from build123d import *

# Parameters (mm, degrees)
SKETCH_2_W             = 126
SKETCH_2_H             = 22
SKETCH_2_R             = 1.7
SM_BASE_FLANGE_1_DEPTH = 2.5
OTHER_START            = -15.764824005
OTHER_1_DEPTH          = 22
OTHER_START_2          = -11.014823905
OTHER_1_2_DEPTH        = 12.4999998
OTHER_1_3_DEPTH        = 1.3499999
OTHER_START_3          = 4.885176095
OTHER_1_4_DEPTH        = 1.3499999
OTHER_START_4          = -14.414824105
OTHER_1_5_DEPTH        = 19.3000002
OTHER_START_5          = -51.7366
OTHER_1_6_OUTLINE_R    = 1.7
OTHER_1_6_DEPTH        = 103.4732
CUT_EXTRUDE_1_DEPTH    = 57.025302757


with BuildPart() as part:
    # 基体-法兰1: sheet metal written as solids
    # Sketch 2 → 基体-法兰1 (new body)
    with BuildSketch(Plane(origin=(0, 0, 0), x_dir=(1, 0, 0), z_dir=(0, 1, 0))):
        with Locations((0, 4.764824005)):
            Rectangle(SKETCH_2_W, SKETCH_2_H)
        with Locations(Location((57.5, 12.714824005, 0), (0, 0, 270))):
            Circle(SKETCH_2_R, mode=Mode.SUBTRACT)
        with Locations(Location((57.5, -3.185175995, 0), (0, 0, 270))):
            Circle(SKETCH_2_R, mode=Mode.SUBTRACT)
        with Locations(Location((-57.5, -3.185175995, 0), (0, 0, 90))):
            Circle(SKETCH_2_R, mode=Mode.SUBTRACT)
        with Locations(Location((-57.5, 12.714824005, 0), (0, 0, 90))):
            Circle(SKETCH_2_R, mode=Mode.SUBTRACT)
    extrude(amount=-SM_BASE_FLANGE_1_DEPTH)

    # Other 1: read off the stored shape, not the designer's step
    # Other 1 outline → Other 1 (cut)
    with BuildSketch(Plane.XY.offset(OTHER_START)):
        with BuildLine():
            Line((-63, -2.5), (-48.5, -2.5))
            ThreePointArc((-48.5, -2.5), (-50.511404982, -1.799110859), (-51.651666226, 0))
            Line((-51.651666226, 0), (-63, 0))
            Line((-63, 0), (-63, -2.5))
        make_face()
        with BuildLine():
            ThreePointArc((51.651666226, 0), (50.511404982, -1.799110859), (48.5, -2.5))
            Line((48.5, -2.5), (63, -2.5))
            Line((63, -2.5), (63, 0))
            Line((63, 0), (51.651666226, 0))
        make_face()
    extrude(amount=OTHER_1_DEPTH, mode=Mode.SUBTRACT)

    # Other 1 2 outline → Other 1 2 (add)
    with BuildSketch(Plane.XY.offset(OTHER_START_2)):
        with BuildLine():
            ThreePointArc((-51.7366, 0.7366), (-51.715296446, 0.365859759), (-51.651666226, 0))
            Line((-51.651666226, 0), (-48.5, 0))
            ThreePointArc((-48.5, 0), (-49.020854855, 0.215745145), (-49.2366, 0.7366))
            Line((-49.2366, 0.7366), (-49.2366, 12.116056017))
            Line((-49.2366, 12.116056017), (-51.7366, 12.116056017))
            Line((-51.7366, 12.116056017), (-51.7366, 0.7366))
        make_face()
        with BuildLine():
            Line((48.5, 0), (51.651666226, 0))
            ThreePointArc((51.651666226, 0), (51.715296446, 0.365859759), (51.7366, 0.7366))
            Line((51.7366, 0.7366), (51.7366, 12.116056017))
            Line((51.7366, 12.116056017), (49.2366, 12.116056017))
            Line((49.2366, 12.116056017), (49.2366, 0.7366))
            ThreePointArc((49.2366, 0.7366), (49.020854855, 0.215745145), (48.5, 0))
        make_face()
    extrude(amount=OTHER_1_2_DEPTH)

    # Other 1 3 outline → Other 1 3 (add)
    with BuildSketch(Plane.XY.offset(OTHER_START)):
        with BuildLine():
            ThreePointArc((-51.7366, 0.7366), (-51.715296446, 0.365859759), (-51.651666226, 0))
            Line((-51.651666226, 0), (-48.5, 0))
            ThreePointArc((-48.5, 0), (-49.020854855, 0.215745145), (-49.2366, 0.7366))
            Line((-49.2366, 0.7366), (-49.2366, 12.116056017))
            Line((-49.2366, 12.116056017), (-51.7366, 12.116056017))
            Line((-51.7366, 12.116056017), (-51.7366, 0.7366))
        make_face()
        with BuildLine():
            Line((48.5, 0), (51.651666226, 0))
            ThreePointArc((51.651666226, 0), (51.715296446, 0.365859759), (51.7366, 0.7366))
            Line((51.7366, 0.7366), (51.7366, 12.116056017))
            Line((51.7366, 12.116056017), (49.2366, 12.116056017))
            Line((49.2366, 12.116056017), (49.2366, 0.7366))
            ThreePointArc((49.2366, 0.7366), (49.020854855, 0.215745145), (48.5, 0))
        make_face()
    extrude(amount=OTHER_1_3_DEPTH)

    # Other 1 4 outline → Other 1 4 (add)
    with BuildSketch(Plane.XY.offset(OTHER_START_3)):
        with BuildLine():
            ThreePointArc((-51.7366, 0.7366), (-51.715296446, 0.365859759), (-51.651666226, 0))
            Line((-51.651666226, 0), (-48.5, 0))
            ThreePointArc((-48.5, 0), (-49.020854855, 0.215745145), (-49.2366, 0.7366))
            Line((-49.2366, 0.7366), (-49.2366, 12.116056017))
            Line((-49.2366, 12.116056017), (-51.7366, 12.116056017))
            Line((-51.7366, 12.116056017), (-51.7366, 0.7366))
        make_face()
        with BuildLine():
            Line((48.5, 0), (51.651666226, 0))
            ThreePointArc((51.651666226, 0), (51.715296446, 0.365859759), (51.7366, 0.7366))
            Line((51.7366, 0.7366), (51.7366, 12.116056017))
            Line((51.7366, 12.116056017), (49.2366, 12.116056017))
            Line((49.2366, 12.116056017), (49.2366, 0.7366))
            ThreePointArc((49.2366, 0.7366), (49.020854855, 0.215745145), (48.5, 0))
        make_face()
    extrude(amount=OTHER_1_4_DEPTH)

    # Other 1 5 outline → Other 1 5 (add)
    with BuildSketch(Plane.XY.offset(OTHER_START_4)):
        with BuildLine():
            ThreePointArc((49.2366, 0.7366), (49.020854855, 0.215745145), (48.5, 0))
            Line((48.5, 0), (51.651666226, 0))
            ThreePointArc((51.651666226, 0), (51.715296446, 0.365859759), (51.7366, 0.7366))
            Line((51.7366, 0.7366), (51.7366, 12.116056017))
            Line((51.7366, 12.116056017), (49.2366, 12.116056017))
            Line((49.2366, 12.116056017), (49.2366, 0.7366))
        make_face()
        with BuildLine():
            ThreePointArc((-51.7366, 0.7366), (-51.715296446, 0.365859759), (-51.651666226, 0))
            Line((-51.651666226, 0), (-48.5, 0))
            ThreePointArc((-48.5, 0), (-49.020854855, 0.215745145), (-49.2366, 0.7366))
            Line((-49.2366, 0.7366), (-49.2366, 12.116056017))
            Line((-49.2366, 12.116056017), (-51.7366, 12.116056017))
            Line((-51.7366, 12.116056017), (-51.7366, 0.7366))
        make_face()
    extrude(amount=OTHER_1_5_DEPTH)

    # Other 1 6 outline → Other 1 6 (cut)
    with BuildSketch(Plane.YZ.offset(OTHER_START_5)):
        with Locations((6.616056017, -12.714824005)):
            Circle(OTHER_1_6_OUTLINE_R)
        with Locations((6.616056017, 3.185175995)):
            Circle(OTHER_1_6_OUTLINE_R)
    extrude(amount=OTHER_1_6_DEPTH, mode=Mode.SUBTRACT)

    # 草图8 → 切除-拉伸1 (cut, through all)
    with BuildSketch(Plane.XZ.offset(2.5)):
        with BuildLine():
            Line((-8, -3.764824005), (8, -3.764824005))
            ThreePointArc((8, -3.764824005), (9, -4.764824005), (8, -5.764824005))
            Line((8, -5.764824005), (-8, -5.764824005))
            ThreePointArc((-8, -5.764824005), (-9, -4.764824005), (-8, -3.764824005))
        make_face()
        with BuildLine():
            Line((-38, -3.764824005), (-22, -3.764824005))
            ThreePointArc((-22, -3.764824005), (-21, -4.764824005), (-22, -5.764824005))
            Line((-22, -5.764824005), (-38, -5.764824005))
            ThreePointArc((-38, -5.764824005), (-39, -4.764824005), (-38, -3.764824005))
        make_face()
        with BuildLine():
            Line((22, -3.764824005), (38, -3.764824005))
            ThreePointArc((38, -3.764824005), (39, -4.764824005), (38, -5.764824005))
            Line((38, -5.764824005), (22, -5.764824005))
            ThreePointArc((22, -5.764824005), (21, -4.764824005), (22, -3.764824005))
        make_face()
        with BuildLine():
            Line((-8, -11.764824005), (8, -11.764824005))
            ThreePointArc((8, -11.764824005), (9, -12.764824005), (8, -13.764824005))
            Line((8, -13.764824005), (-8, -13.764824005))
            ThreePointArc((-8, -13.764824005), (-9, -12.764824005), (-8, -11.764824005))
        make_face()
        with BuildLine():
            Line((-38, -11.764824005), (-22, -11.764824005))
            ThreePointArc((-22, -11.764824005), (-21, -12.764824005), (-22, -13.764824005))
            Line((-22, -13.764824005), (-38, -13.764824005))
            ThreePointArc((-38, -13.764824005), (-39, -12.764824005), (-38, -11.764824005))
        make_face()
        with BuildLine():
            Line((22, -11.764824005), (38, -11.764824005))
            ThreePointArc((38, -11.764824005), (39, -12.764824005), (38, -13.764824005))
            Line((38, -13.764824005), (22, -13.764824005))
            ThreePointArc((22, -13.764824005), (21, -12.764824005), (22, -11.764824005))
        make_face()
        with BuildLine():
            Line((-8, 4.235175995), (8, 4.235175995))
            ThreePointArc((8, 4.235175995), (9, 3.235175995), (8, 2.235175995))
            Line((8, 2.235175995), (-8, 2.235175995))
            ThreePointArc((-8, 2.235175995), (-9, 3.235175995), (-8, 4.235175995))
        make_face()
        with BuildLine():
            Line((-38, 4.235175995), (-22, 4.235175995))
            ThreePointArc((-22, 4.235175995), (-21, 3.235175995), (-22, 2.235175995))
            Line((-22, 2.235175995), (-38, 2.235175995))
            ThreePointArc((-38, 2.235175995), (-39, 3.235175995), (-38, 4.235175995))
        make_face()
        with BuildLine():
            Line((22, 4.235175995), (38, 4.235175995))
            ThreePointArc((38, 4.235175995), (39, 3.235175995), (38, 2.235175995))
            Line((38, 2.235175995), (22, 2.235175995))
            ThreePointArc((22, 2.235175995), (21, 3.235175995), (22, 4.235175995))
        make_face()
        with BuildLine():
            Line((-25, 0.235175995), (-5, 0.235175995))
            ThreePointArc((-5, 0.235175995), (-4, -0.764824005), (-5, -1.764824005))
            Line((-5, -1.764824005), (-25, -1.764824005))
            ThreePointArc((-25, -1.764824005), (-26, -0.764824005), (-25, 0.235175995))
        make_face()
        with BuildLine():
            Line((5, 0.235175995), (25, 0.235175995))
            ThreePointArc((25, 0.235175995), (26, -0.764824005), (25, -1.764824005))
            Line((25, -1.764824005), (5, -1.764824005))
            ThreePointArc((5, -1.764824005), (4, -0.764824005), (5, 0.235175995))
        make_face()
        with BuildLine():
            Line((-25, -7.764824005), (-5, -7.764824005))
            ThreePointArc((-5, -7.764824005), (-4, -8.764824005), (-5, -9.764824005))
            Line((-5, -9.764824005), (-25, -9.764824005))
            ThreePointArc((-25, -9.764824005), (-26, -8.764824005), (-25, -7.764824005))
        make_face()
        with BuildLine():
            Line((5, -7.764824005), (25, -7.764824005))
            ThreePointArc((25, -7.764824005), (26, -8.764824005), (25, -9.764824005))
            Line((25, -9.764824005), (5, -9.764824005))
            ThreePointArc((5, -9.764824005), (4, -8.764824005), (5, -7.764824005))
        make_face()
    extrude(amount=-CUT_EXTRUDE_1_DEPTH, mode=Mode.SUBTRACT)


solid = part.part
Input: part model. Units: mm. Frame: model coordinates. A direction names the side the tool comes from. Coordinates: 2 decimals unless noted, no trailing zeros. Order: outer loops, then holes, each group sorted by start corner. A loop starts at its lowest first (then second) coordinate and runs counter-clockwise, first axis right, second up. Notation, with made-up numbers: M 60.5,36 L 114.5,36 A22 cw 114.5,74 Z; hole C 87,85.5 d8. An arc over 180 degrees is marked long. One line per question, with ' | ' between items.
Item 1: Section B-B (x = -32). Output: boundary loops of the cut face in (y, z).
Geometry results:
outline: M -2.5,-15.76 L 0,-15.76 L 0,-13.76 L -2.5,-13.76 Z; M -2.5,-11.76 L 0,-11.76 L 0,-5.76 L -2.5,-5.76 Z; M -2.5,-3.76 L 0,-3.76 L 0,2.24 L -2.5,2.24 Z; M -2.5,4.24 L 0,4.24 L 0,6.24 L -2.5,6.24 Z
Item 2: Pin query (flat end, axial travel): pin 1 (6 mm diameter, centred on x = -35, y = 4.5, fed in from -Z); pin 2 (6 mm diameter, centred on x = 9.5, z = -11, fed in from +Y). Return the tip coordinate at first contact, or that it passes through.
Geometry results:
pin 1: passes through | pin 2: stops at y = 0
Item 3: Reachability of faces 1 (the cylindrical face through (-50.81, -1.53, -4.92)), 2 (the cylindrical face through (26, -1.27, -0.74)), 3 (the flat face through (-49.237, 6, -5)) from +Z, -Z, +X, -X, +Y, -Y: full face, straight path, thin tool, end or side. Return the list, or none.
Geometry results:
face 1: +Z, -Z, -X, -Y | face 2: +Y, -Y | face 3: +Z, -Z, +Y
Item 4: Ray query, line 1 along X through (y, z) = (3.5, -3); line 2 along Y through (x, z) = (-17, -12); line 3 along X through (y, z) = (0.25, -10.5). Return the intervals inside material, ascending.
Geometry results:
line 1: x = -51.74 to -49.24, 49.24 to 51.74 | line 2: y = -2.5 to 0 | line 3: x = -51.7 to -49.05, 49.05 to 51.7
Item 5: Draft query along Y for faces 4 (the cylindrical face through (21, -1.3, -12.8)), 5 (the flat face through (-50, 12.116, -5)), 6 (the cylindrical face through (50.469, 7.401, -14.223)). Return one class per face: released by +Y, released by -Y, zero draft, split by the parting line, or undercut.
Geometry results:
face 4: zero draft | face 5: released by +Y | face 6: undercut
Item 6: Section C-C (z = -8.75). Output: boundary loops of the cut face in (x, y).
Geometry results:
outline: M -51.74,0.74 A3.24 ccw -48.5,-2.5 L -26,-2.5 L -26,0 L -48.5,0 A0.74 cw -49.24,0.74 L -49.24,12.12 L -51.74,12.12 Z; M -4,-2.5 L 4,-2.5 L 4,0 L -4,0 Z; M 26,-2.5 L 48.5,-2.5 A3.24 ccw 51.74,0.74 L 51.74,12.12 L 49.24,12.12 L 49.24,0.74 A0.74 cw 48.5,0 L 26,0 Z
Item 7: Section D-D (x = 44). Output: boundary loops of the cut face in (y, z).
Geometry results:
outline: M -2.5,-15.76 L 0,-15.76 L 0,6.24 L -2.5,6.24 Z
Item 8: Section A-A (y = 3.25). Output: boundary loops of the cut face in (x, z), then the cut area to 3 significant figures.
Geometry results:
outline: M -51.74,-15.76 L -49.24,-15.76 L -49.24,6.24 L -51.74,6.24 Z; M 49.24,-15.76 L 51.74,-15.76 L 51.74,6.24 L 49.24,6.24 Z | area: 110 mm^2
